from build123d import *

# Parameters (mm, degrees)
ESQUISSE1_R             = 13.075
BOSS_EXTRU_1_DEPTH      = 65.7
ESQUISSE2_R             = 10.075
ENL_V_MAT_EXTRU_1_DEPTH = 0.1
ESQUISSE3_R             = 8.575
ESQUISSE3_R_2           = 7.075
ENL_V_MAT_EXTRU_2_DEPTH = 2


with BuildPart() as part:
    # Esquisse1 → Boss.-Extru.1 (new body)
    with BuildSketch(Plane(origin=(0, 0, 0), x_dir=(1, 0, 0), z_dir=(0, 1, 0))):
        Circle(ESQUISSE1_R)
    extrude(amount=BOSS_EXTRU_1_DEPTH)

    # Esquisse2 → Enlèv. mat.-Extru.1 (cut)
    with BuildSketch(Plane(origin=(0, 65.7, 0), x_dir=(1, 0, 0), z_dir=(0, 1, 0))):
        Circle(ESQUISSE2_R)
    extrude(amount=-ENL_V_MAT_EXTRU_1_DEPTH, mode=Mode.SUBTRACT)

    # Esquisse3 → Enlèv. mat.-Extru.2 (cut)
    with BuildSketch(Plane.XZ):
        Circle(ESQUISSE3_R)
        Circle(ESQUISSE3_R_2, mode=Mode.SUBTRACT)
    extrude(amount=-ENL_V_MAT_EXTRU_2_DEPTH, mode=Mode.SUBTRACT)


solid = part.part
The listing builds one solid part. Answer for the finished solid, in the listing's coordinates (mm). A direction names the side the tool comes from. Give positions to 0.01 mm unless a question says otherwise; leave off trailing zeros. Write each loop counter-clockwise with the first axis right and the second up, starting at its lowest first coordinate (ties: lowest second). Pieces come first, ordered by that corner, then holes.
1) Section B-B (z = -5.25) is taken. Write down the section's boundary in (x, y).
2) Section C-C (y = 34) is taken. Write down the section's boundary in (x, z) (3 decimals).
3) Section D-D (x = -7.75) is taken. Write down the section's boundary in (y, z), and give its area (3 significant figures).
4) Find the intervals of material crossed by L1, parallel to Z at x = 0, y = 1.55 (3 decimals); L2, parallel to Z at x = 0, y = 65.65 (3 decimals); L3, parallel to Y at x = 5, z = -2.25, in increasing order.
5) Section A-A (x = 4.75) is taken. Write down the section's boundary in (y, z) (3 decimals).
6) For a pull along Z with two mould halves and no side action, classify faces 4 (the face through (0, 0, 0)), 5 (the face through (-2.834, 32.39, 12.764)), 6 (the face through (3.26, 0.99, -6.28)) as pulls with the +Z half, pulls with the -Z half, needs draft (parallel to the pull), parting line crosses it, or undercut.
7) A tool of negligible diameter and unlimited length cuts with its end or side. For faces 1 (the face through (0, 65.6, 0)), 2 (the face through (8.179, 0.986, 2.576)), 3 (the face through (3, 0, 9)), from which of +Z, -Z, +X, -X, +Y, -Y can it reach the whole face along a straight path? Write none if from no direction.
8) Given P1, Ø6, axis at y = 52, z = -6.5, coming from the -X side; P2, Ø6, axis at x = -7.5, y = 40, coming from the +Z side; P3, Ø1, axis at y = 49.5, z = -1, coming from the +X side, each flat-ended and moving along its own axis, determine where each tip first touches the part or whether it passes through.
Response:
1. outline: (-11.97, 0) - (-6.78, 0) - (-6.78, 2) - (-4.74, 2) - (-4.74, 0) - (4.74, 0) - (4.74, 2) - (6.78, 2) - (6.78, 0) - (11.97, 0) - (11.97, 65.7) - (8.6, 65.7) - (8.6, 65.6) - (-8.6, 65.6) - (-8.6, 65.7) - (-11.97, 65.7) - close
2. outline: circle Ø26.15 at (0, 0)
3. outline: (0, -10.53) - (65.7, -10.53) - (65.7, -6.44) - (65.6, -6.44) - (65.6, 6.44) - (65.7, 6.44) - (65.7, 10.53) - (0, 10.53) - (0, 3.67) - (2, 3.67) - (2, -3.67) - (0, -3.67) - close
3. area: 1,370 mm2
4. L1: z = -13.075 to -8.575, -7.075 to 7.075, 8.575 to 13.075
4. L2: z = -13.075 to -10.075, 10.075 to 13.075
4. L3: y = 0 to 65.6
5. outline: (0, -12.182) - (65.7, -12.182) - (65.7, -8.885) - (65.6, -8.885) - (65.6, 8.885) - (65.7, 8.885) - (65.7, 12.182) - (0, 12.182) - (0, 7.139) - (2, 7.139) - (2, 5.243) - (0, 5.243) - (0, -5.243) - (2, -5.243) - (2, -7.139) - (0, -7.139) - close
6. face 4: needs draft
6. face 5: parting line crosses it
6. face 6: undercut
7. face 1: +Y
7. face 2: -Y
7. face 3: +Z, -Z, +X, -X, -Y
8. P1: stops at x = -12.6
8. P2: stops at z = 12.28
8. P3: stops at x = 13.07
